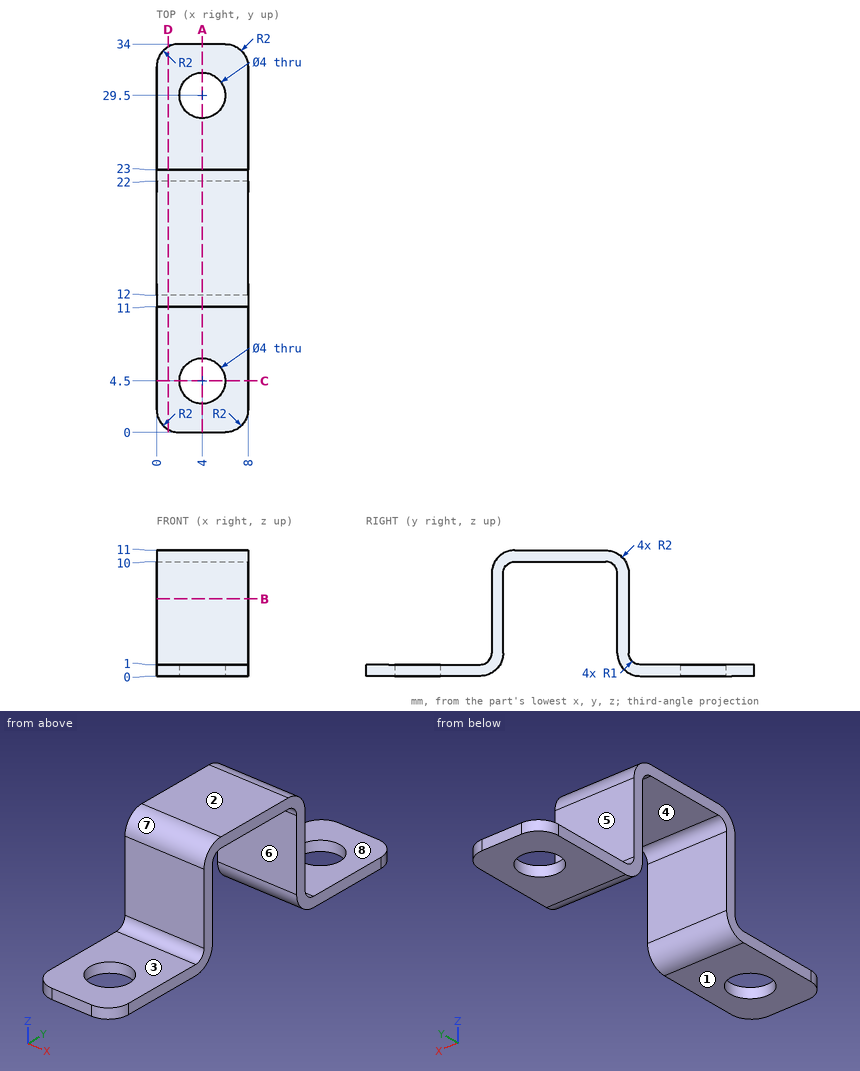
The drawing under review shows one solid part. Ordinate dimensions are in mm from its lowest x, y, z. A direction names the side the tool comes from. Coordinates: 2 decimals unless noted, no trailing zeros. Order: outer loops, then holes, each group sorted by start corner. A loop starts at its lowest first (then second) coordinate and runs counter-clockwise, first axis right, second up. Notation, with made-up numbers: (8, 55) -> (34, 55) arc R20 cw to (34, 70) -> close; hole circle Ø11 at (-7, 75.5). An arc over 180 degrees is marked (long way). Answer in a Markdown table with one row per item.
(1) Machinability: for the marked faces 1, 2, 3, 4 and 5, which of the approach directions +Z, -Z, +X, -X, +Y, -Y give a long, thin tool a straight path to every point of the face, cutting with its end or side? Answer none if there is none.
Answers:
| item | result |
|---|---|
| face 1 | -Z, +X, -X, +Y, -Y |
| face 2 | +Z, +X, -X, +Y, -Y |
| face 3 | +Z, +X, -X, -Y |
| face 4 | -Z, +X, -X |
| face 5 | +Z, +X, -X, +Y |
(2) Consider section D-D (x = 1). Write out the cut boundary in (y, z), plus the area to 3 significant figures.
Answers:
| item | result |
|---|---|
| outline | (0.27, 0) -> (10, 0) arc R2 ccw to (12, 2) -> (12, 9) arc R1 cw to (13, 10) -> (21, 10) arc R1 cw to (22, 9) -> (22, 2) arc R2 ccw to (24, 0) -> (33.73, 0) -> (33.73, 1) -> (24, 1) arc R1 cw to (23, 2) -> (23, 9) arc R2 ccw to (21, 11) -> (13, 11) arc R2 ccw to (11, 9) -> (11, 2) arc R1 cw to (10, 1) -> (0.27, 1) -> close |
| area | 50.9 mm² |
(3) Consider section A-A (x = 4). Write out the cut boundary in (y, z).
Answers:
| item | result |
|---|---|
| outline | (0, 0) -> (2.5, 0) -> (2.5, 1) -> (0, 1) -> close; (6.5, 0) -> (10, 0) arc R2 ccw to (12, 2) -> (12, 9) arc R1 cw to (13, 10) -> (21, 10) arc R1 cw to (22, 9) -> (22, 2) arc R2 ccw to (24, 0) -> (27.5, 0) -> (27.5, 1) -> (24, 1) arc R1 cw to (23, 2) -> (23, 9) arc R2 ccw to (21, 11) -> (13, 11) arc R2 ccw to (11, 9) -> (11, 2) arc R1 cw to (10, 1) -> (6.5, 1) -> close; (31.5, 0) -> (34, 0) -> (34, 1) -> (31.5, 1) -> close |
(4) Wall thickness on line 1 along Y through (x, z) = (4.5, 6); line 2 along Y through (x, z) = (4, 0.8); line 3 along Z through (x, y) = (5, 14): over which ranges is each line inside the solid? List them lowest first.
Answers:
| item | result |
|---|---|
| line 1 | 11 to 12, 22 to 23 |
| line 2 | 0 to 2.5, 6.5 to 11.6, 22.4 to 27.5, 31.5 to 34 |
| line 3 | 10 to 11 |
(5) Insertion check: pin 1 (1.5 mm diameter, centred on x = 5, y = 28.5, fed in from +Z); pin 2 (2 mm diameter, centred on x = 2, z = 5, fed in from +Y); pin 3 (3.5 mm diameter, centred on x = 4.5, z = 7, fed in from -Y). Each pin has a flat end and moves straight along its axis. Give the tip position at first contact, or say it passes through.
Answers:
| item | result |
|---|---|
| pin 1 | z = 1 |
| pin 2 | y = 23 |
| pin 3 | y = 11 |
(6) The part is to be moulded in two halves that separate along Y. For the marked faces 6, 7 and 8, say which applies: +Y half, -Y half, draft (parallel to the pull), parting line (faces both ways), or undercut.
Answers:
| item | result |
|---|---|
| face 6 | undercut |
| face 7 | -Y half |
| face 8 | draft |
(7) Consider section C-C (y = 4.5). Write out the cut boundary in (x, z), plus the area to 3 significant figures.
Answers:
| item | result |
|---|---|
| outline | (0, 0) -> (2, 0) -> (2, 1) -> (0, 1) -> close; (6, 0) -> (8, 0) -> (8, 1) -> (6, 1) -> close |
| area | 4.00 mm² |
(8) Consider section B-B (z = 6.75). Write out the cut boundary in (x, y).
Answers:
| item | result |
|---|---|
| outline | (0, 11) -> (8, 11) -> (8, 12) -> (0, 12) -> close; (0, 22) -> (8, 22) -> (8, 23) -> (0, 23) -> close |
